```python
from build123d import *

# Parameters (mm, degrees)
SKETCH1_R           = 45.72
BOSS_EXTRUDE1_DEPTH = 12.7
SKETCH2_R           = 33.02
BOSS_EXTRUDE2_DEPTH = 120.65
SKETCH3_R           = 25.4
CUT_EXTRUDE1_DEPTH  = 128.27
SKETCH4_R           = 2.54
CUT_EXTRUDE2_DEPTH  = 128.27
SKETCH5_R           = 3.175
CUT_EXTRUDE3_DEPTH  = 128.27
SKETCH6_R           = 10.16
CUT_EXTRUDE4_DEPTH  = 0.127
CIRPATTERN1_COUNT   = 16
SKETCH7_R           = 1.7526
CUT_EXTRUDE5_DEPTH  = 144.644803944
CIRPATTERN2_COUNT   = 4


with BuildPart() as part:
    # Sketch1 → Boss-Extrude1 (new body)
    with BuildSketch(Plane(origin=(0, 0, 0), x_dir=(1, 0, 0), z_dir=(0, 1, 0))):
        with Locations(Location((0, 0, 0), (0, 0, 270))):
            Circle(SKETCH1_R)
    extrude(amount=BOSS_EXTRUDE1_DEPTH)

    # Sketch2 → Boss-Extrude2 (add)
    with BuildSketch(Plane(origin=(0, 12.7, 0), x_dir=(1, 0, 0), z_dir=(0, 1, 0))):
        with Locations(Location((0, 0, 0), (0, 0, 90))):
            Circle(SKETCH2_R)
    extrude(amount=BOSS_EXTRUDE2_DEPTH)

    # Sketch3 → Cut-Extrude1 (cut)
    with BuildSketch(Plane.XZ):
        with Locations(Location((0, 0, 0), (0, 0, 270))):
            Circle(SKETCH3_R)
    extrude(amount=-CUT_EXTRUDE1_DEPTH, mode=Mode.SUBTRACT)

    # Sketch4 → Cut-Extrude2 (cut)
    with BuildSketch(Plane(origin=(0, 133.35, 0), x_dir=(1, 0, 0), z_dir=(0, 1, 0))):
        with Locations(Location((0, 0, 0), (0, 0, 270))):
            Circle(SKETCH4_R)
    extrude(amount=-CUT_EXTRUDE2_DEPTH, mode=Mode.SUBTRACT)

    # Sketch5 → Cut-Extrude3 (cut)
    with BuildSketch(Plane.XZ):
        with Locations(Location((-13.759658147, -38.23978828, 0), (0, 0, 270))):
            Circle(SKETCH5_R)
    cut_extrude3 = extrude(amount=-CUT_EXTRUDE3_DEPTH, mode=Mode.SUBTRACT)

    # Sketch6 → Cut-Extrude4 (cut)
    with BuildSketch(Plane.XZ.offset(-128.27)):
        with Locations(Location((0, 0, 0), (0, 0, 270))):
            Circle(SKETCH6_R)
    extrude(amount=-CUT_EXTRUDE4_DEPTH, mode=Mode.SUBTRACT)

    # CirPattern1: Cut-Extrude3 ×16 about axis
    cirpattern1_axis = Axis((0, 0, 0), (0, 1, 0))
    for i in range(1, CIRPATTERN1_COUNT):
        add(cut_extrude3.rotate(cirpattern1_axis, i * 360 / CIRPATTERN1_COUNT), mode=Mode.SUBTRACT)

    # Sketch7 → Cut-Extrude5 (cut, through all)
    with BuildSketch(Plane.XZ.offset(-128.27)):
        with Locations(Location((13.208, 0, 0), (0, 0, 270))):
            Circle(SKETCH7_R)
    cut_extrude5 = extrude(amount=-CUT_EXTRUDE5_DEPTH, mode=Mode.SUBTRACT)

    # CirPattern2: Cut-Extrude5 ×4 about axis
    cirpattern2_axis = Axis((0, 0, 0), (0, 1, 0))
    for i in range(1, CIRPATTERN2_COUNT):
        add(cut_extrude5.rotate(cirpattern2_axis, i * 360 / CIRPATTERN2_COUNT), mode=Mode.SUBTRACT)


solid = part.part
```
CAD build for the part. Positions are in the model's coordinates, mm. A direction names the side the tool comes from. Coordinates: 2 decimals unless noted, no trailing zeros. Write each loop counter-clockwise with the first axis right and the second up, starting at its lowest first coordinate (ties: lowest second). Pieces come first, ordered by that corner, then holes.
(1) Flat gauge pins, fed straight in: pin 1 (2 mm diameter, centred on x = 0, z = 13.208, fed in from +Y); pin 2 (10 mm diameter, centred on x = -1, y = 70.5, fed in from -Z); pin 3 (3 mm diameter, centred on y = 62, z = -10.5, fed in from -X); pin 4 (7.5 mm diameter, centred on x = -36.77, z = -17.31, fed in from +Y). Where does each tip first touch, or does it go through?
(2) Drill centre lines: probe 1 along X at (y, z) = (129.55, 0); probe 2 along Z at (x, y) = (0.5, 68); probe 3 along Z at (x, y) = (29, 10). Where is each one in solid material? Low to high.
(3) Two-plate mould, pull along X, no slides. Class faces 3 (the face through (20.1, 72.2, 26.2)), 4 (the face through (7, 133.35, 0)), 5 (the face through (-17.173, 6.261, 33.597)): +X half, -X half, draft (parallel to the pull), parting line (faces both ways), or undercut.
(4) Cut at A-A, the plane y = 50. List the corners of the cut face in (x, z), and give its area (3 significant figures).
(5) Cut at B-B, the plane z = 8. List the corners of the cut face in (x, y), and give its area (3 significant figures).
(6) 3-axis set-ups, long thin cutter, end or side, ignore diameter. For faces 1 (the face through (-14.946, 130.774, -0.228)), 2 (the face through (0, 128.27, -11)): which of +Z, -Z, +X, -X, +Y, -Y reach the whole face in a straight line?
Geometry says:
1. pin 1: passes through
1. pin 2: stops at z = -33.02
1. pin 3: stops at x = -31.77
1. pin 4: stops at y = 12.7
2. probe 1: x = -33.02 to -14.96, -11.46 to -2.54, 2.54 to 11.46, 14.96 to 33.02
2. probe 2: z = -33.02 to -25.4, 25.4 to 33.02
2. probe 3: z = -35.35 to -30.34, -24.35 to 27.35, 32.77 to 35.35
3. face 3: parting line
3. face 4: draft
3. face 5: undercut
4. outline: circle Ø66.04 at (0, 0); hole circle Ø50.8 at (0, 0)
4. area: 1,400 mm2
5. outline: (-45.01, 0) - (-24.11, 0) - (-24.11, 128.27) - (-6.26, 128.27) - (-6.26, 128.4) - (6.26, 128.4) - (6.26, 128.27) - (24.11, 128.27) - (24.11, 0) - (45.01, 0) - (45.01, 12.7) - (32.04, 12.7) - (32.04, 133.35) - (-32.04, 133.35) - (-32.04, 12.7) - (-45.01, 12.7) - close
5. area: 2,690 mm2
6. face 1: +Y, -Y
6. face 2: -Y
